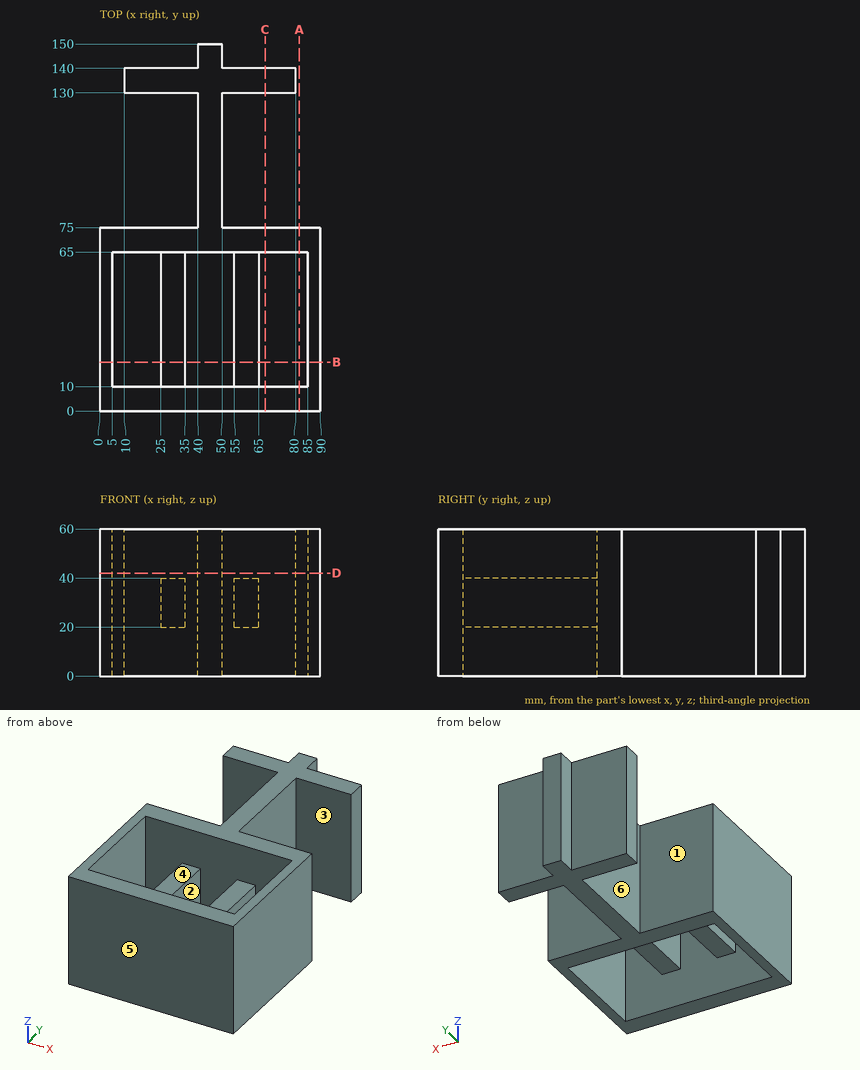
Here's the drawing with two shaded views (mm, measured from the low corner). I have some questions. A direction names the side the tool comes from. Coordinates: 2 decimals unless noted, no trailing zeros. Write each loop counter-clockwise with the first axis right and the second up, starting at its lowest first coordinate (ties: lowest second). Pieces come first, ordered by that corner, then holes. Notation, with made-up numbers: (4.5, -26.5) -> (42.5, -26.5) arc R15 ccw to (42.5, -14.5) -> close; hole circle Ø11 at (32.25, 76.25). An arc over 180 degrees is marked (long way). Use a Markdown table: item, result. Add a question column.
(1) We'd pull the mould along X, two halves only. Please class the marked faces 4, 5 and 6: +X half, -X half, draft (parallel to the pull), parting line (faces both ways), or undercut.
(2) If we section it at D-D, the plane z = 42: Write out the boundary of the cut face in (x, y).
(3) If we section it at B-B, the plane y = 20: Write out the boundary of the cut face in (x, z), and give its area (3 significant figures).
(4) For the marked faces 1, 2 and 3, which set-ups out of +Z, -Z, +X, -X, +Y, -Y let a thin tool reach every point of the face, with its end or its side?
(5) If we section it at C-C, the plane x = 67.5: Write out the boundary of the cut face in (y, z), and give its area (3 significant figures).
(6) Please list where these lines run through material, in increasing order: line 1 (Y direction, x = 75, z = 15.5); line 2 (X direction, y = 23.5, z = 35); line 3 (Y direction, x = 27, z = 23).
(7) If we section it at A-A, the plane x = 81.5: Write out the boundary of the cut face in (y, z).
(8) I'm going to push flat-ended pins straight in: P1, Ø3, axis at y = 145, z = 35, coming from the +X side; P2, Ø11, axis at x = 62, y = 42, coming from the +Z side; P3, Ø1.5, axis at x = 77.5, z = 6, coming from the +Y side. Where does each tip first touch, or does it pass through?
Outcome:
| question | item | result |
|---|---|---|
| 1 | face 4 | undercut |
| 1 | face 5 | draft |
| 1 | face 6 | -X half |
| 2 | outline | (0, 0) -> (90, 0) -> (90, 75) -> (50, 75) -> (50, 130) -> (80, 130) -> (80, 140) -> (50, 140) -> (50, 150) -> (40, 150) -> (40, 140) -> (10, 140) -> (10, 130) -> (40, 130) -> (40, 75) -> (0, 75) -> close; hole (5, 10) -> (85, 10) -> (85, 65) -> (5, 65) -> close |
| 3 | outline | (0, 0) -> (5, 0) -> (5, 60) -> (0, 60) -> close; (25, 20) -> (35, 20) -> (35, 40) -> (25, 40) -> close; (55, 20) -> (65, 20) -> (65, 40) -> (55, 40) -> close; (85, 0) -> (90, 0) -> (90, 60) -> (85, 60) -> close |
| 3 | area | 1,000 mm^2 |
| 4 | face 1 | +Z, -Z, -X |
| 4 | face 2 | +Z, -Z |
| 4 | face 3 | +Z, -Z, +X |
| 5 | outline | (0, 0) -> (10, 0) -> (10, 60) -> (0, 60) -> close; (65, 0) -> (75, 0) -> (75, 60) -> (65, 60) -> close; (130, 0) -> (140, 0) -> (140, 60) -> (130, 60) -> close |
| 5 | area | 1,800 mm^2 |
| 6 | line 1 | y = 0 to 10, 65 to 75, 130 to 140 |
| 6 | line 2 | x = 0 to 5, 25 to 35, 55 to 65, 85 to 90 |
| 6 | line 3 | y = 0 to 75, 130 to 140 |
| 7 | outline | (0, 0) -> (10, 0) -> (10, 60) -> (0, 60) -> close; (65, 0) -> (75, 0) -> (75, 60) -> (65, 60) -> close |
| 8 | P1 | stops at x = 50 |
| 8 | P2 | stops at z = 40 |
| 8 | P3 | stops at y = 140 |
